Build history of the part. All positions in model axes, mm. Face numbers are marked on the shaded views. A direction names the side the tool comes from. Round coordinates to 2 decimals unless told otherwise and drop trailing zeros. Write each loop counter-clockwise with the first axis right and the second up, starting at its lowest first coordinate (ties: lowest second). Pieces come first, ordered by that corner, then holes. Notation, with made-up numbers: (73.5, 33.25) -> (110.5, 33.25) arc R23 cw to (110.5, 71.25) -> close; hole circle Ø5 at (44.25, -27.75). An arc over 180 degrees is marked (long way). One line per question, with ' | ' between items.
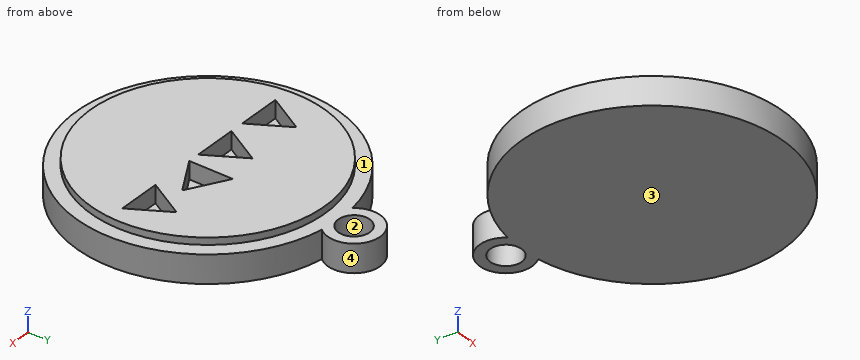
from build123d import *

# Parameters (mm, degrees)
F0_R     = 17.018
F0_R_2   = 2.286
F1_DEPTH = 4.064
F2_DEPTH = 5.08
F4_DEPTH = 2.54


with BuildPart() as f1:
    # F0 (on Top) → F1 (new body)
    with BuildSketch(Plane.XY):
        with BuildLine():
            ThreePointArc((-2.910637, 27.594249), (0, -10.282081), (2.910637, 27.594249))
            ThreePointArc((2.910637, 27.594249), (0, 33.862762), (-2.910637, 27.594249))
        make_face()
        with Locations((0, 8.767919)):
            Circle(F0_R, mode=Mode.SUBTRACT)
        with Locations((0, 30.052762)):
            Circle(F0_R_2, mode=Mode.SUBTRACT)
    extrude(amount=F1_DEPTH)

    # F0 (on Top) → F2 (join)
    with BuildSketch(Plane.XY):
        with Locations((0, 8.767919)):
            Circle(F0_R)
    extrude(amount=F2_DEPTH)

    # F3 (on face) → F4 (cut)
    with BuildSketch(Plane.XY.offset(5.08)):
        Polygon((-8.239756, 7.464734), (-11.410307, 12.945793), (-14.571768, 7.459487), align=None)
        Polygon((0.124255, 7.469981), (-3.046295, 12.95104), (-6.207756, 7.464734), align=None)
        Polygon((1.823385, 7.469981), (7.304444, 10.640532), (1.818137, 13.801993), align=None)
        Polygon((14.575767, 7.475229), (11.405217, 12.956288), (8.243755, 7.469981), align=None)
    extrude(amount=-F4_DEPTH, mode=Mode.SUBTRACT)


solid = f1.part
(1) Slice it at D-D (y = 0). Write the cut outline in (x, z).
Calculated:
outline: (-16.91, 0) -> (16.91, 0) -> (16.91, 4.06) -> (14.59, 4.06) -> (14.59, 5.08) -> (-14.59, 5.08) -> (-14.59, 4.06) -> (-16.91, 4.06) -> close
(2) Drop flat-ended pins along their axis: pin 1 (1.5 mm diameter, centred on x = 11.5, z = 4, fed in from +Y); pin 2 (2.5 mm diameter, centred on x = -3.5, y = 9.5, fed in from +Z); pin 3 (2 mm diameter, centred on y = 16.5, z = 4, fed in from -X). Give the stop position or say it passes through.
Calculated:
pin 1: y = 24.49 | pin 2: z = 2.54 | pin 3: x = -17.82
(3) Mould opens along Y. For the marked faces 3 and 4 say: pulls with the +Y half, pulls with the -Y half, needs draft (parallel to the pull), parting line crosses it, or undercut.
Calculated:
face 3: needs draft | face 4: undercut
(4) Slice it at A-A (x = -0.5). Write the cut outline in (y, z), then the cut area to 3 significant figures.
Calculated:
outline: (-10.28, 0) -> (27.82, 0) -> (27.82, 4.06) -> (25.78, 4.06) -> (25.78, 5.08) -> (8.55, 5.08) -> (8.55, 2.54) -> (7.47, 2.54) -> (7.47, 5.08) -> (-8.24, 5.08) -> (-8.24, 4.06) -> (-10.28, 4.06) -> close; (32.28, 0) -> (33.83, 0) -> (33.83, 4.06) -> (32.28, 4.06) -> close | area: 193 mm2
(5) Slice it at C-C (x = -5.5). Write the cut outline in (y, z), then the cut area to 3 significant figures.
Calculated:
outline: (-9.47, 0) -> (27.01, 0) -> (27.01, 4.06) -> (24.87, 4.06) -> (24.87, 5.08) -> (8.69, 5.08) -> (8.69, 2.54) -> (7.47, 2.54) -> (7.47, 5.08) -> (-7.34, 5.08) -> (-7.34, 4.06) -> (-9.47, 4.06) -> close | area: 178 mm2
(6) Wall check: line 1 (X direction, y = 9.5, z = 4.55); line 2 (Y direction, x = 0, z = 1.85); line 3 (Z direction, x = 10.5, y = -7). Give the ranges that are in metal, low to high. Write a range as from..to.
Calculated:
line 1: -17..-13.4, -9.42..-5.03, -1.05..1.82, 5.33..9.41, 13.4..17 | line 2: -10.28..27.77, 32.34..33.86 | line 3: 0..4.06
(7) 3-axis set-ups, long thin cutter, end or side, ignore diameter. For the marked faces 1 and 2: which of +Z, -Z, +X, -X, +Y, -Y reach the whole face in a straight line?
Calculated:
face 1: +Z | face 2: +Z, -Z
(8) Slice it at B-B (z = 4.55). Write the cut outline in (x, y), then the cut area to 3 significant figures.
Calculated:
outline: circle Ø34.04 at (0, 8.77); hole (-14.57, 7.46) -> (-8.24, 7.46) -> (-11.41, 12.95) -> close; hole (-6.21, 7.46) -> (0.12, 7.47) -> (-3.05, 12.95) -> close; hole (1.82, 7.47) -> (7.3, 10.64) -> (1.82, 13.8) -> close; hole (8.24, 7.47) -> (14.58, 7.48) -> (11.41, 12.96) -> close | area: 840 mm2
